Check sheet for the drawn part. Datum: minimum x, y, z corner. Units: mm. A direction names the side the tool comes from. Coordinates: 2 decimals unless noted, no trailing zeros. Order: outer loops, then holes, each group sorted by start corner. A loop starts at its lowest first (then second) coordinate and runs counter-clockwise, first axis right, second up. Notation, with made-up numbers: M 51,58.5 L 75,58.5 A30 cw 75,85.5 Z; hole C 24.25,-29.75 d9. An arc over 180 degrees is marked long. Return JSON: item names as keys, results as strings. Group by question number.
Q1. Go/stop test with flat-tipped pins: pin 1 Ø4 at (y, z) = (32.5, 13) entering from -X; pin 2 Ø0.8 at (x, y) = (30.5, 20.5) entering from -Z; pin 3 Ø8 at (x, y) = (33.5, 28.5) entering from +Z; pin 4 Ø3 at (y, z) = (23, 14) entering from +X. Record where each tip stops, or that it passes through.
Q2. Section check B-B, the plane x = 21. Enter the section's corners in (y, z).
Q3. Thickness scan on probe 1 along Y at (x, z) = (21, 20.4); probe 2 along Z at (x, y) = (12, 25); probe 3 along Y at (x, z) = (25.5, 4). Record the ranges inside material, lowest first.
Q4. Access from +Z, -Z, +X, -X, +Y, -Y to the whole of each face (thin tool, end or side, straight path). Record for the marked faces 1 and 2.
Q5. Section check D-D, the plane z = 9.5. Enter the section's corners in (x, y), then the cut area to 3 significant figures.
Q6. Mould release check, pull along X, two halves, no side actions. Record for the marked faces 3, 4 and 5: pulls with the +X half, pulls with the -X half, needs draft (parallel to the pull), parting line crosses it, or undercut.
Q7. Section check C-C, the plane y = 21. Enter the section's corners in (x, z).
Q8. Section check A-A, the plane z = 1.75. Enter the section's corners in (x, y), then the cut area to 3 significant figures.
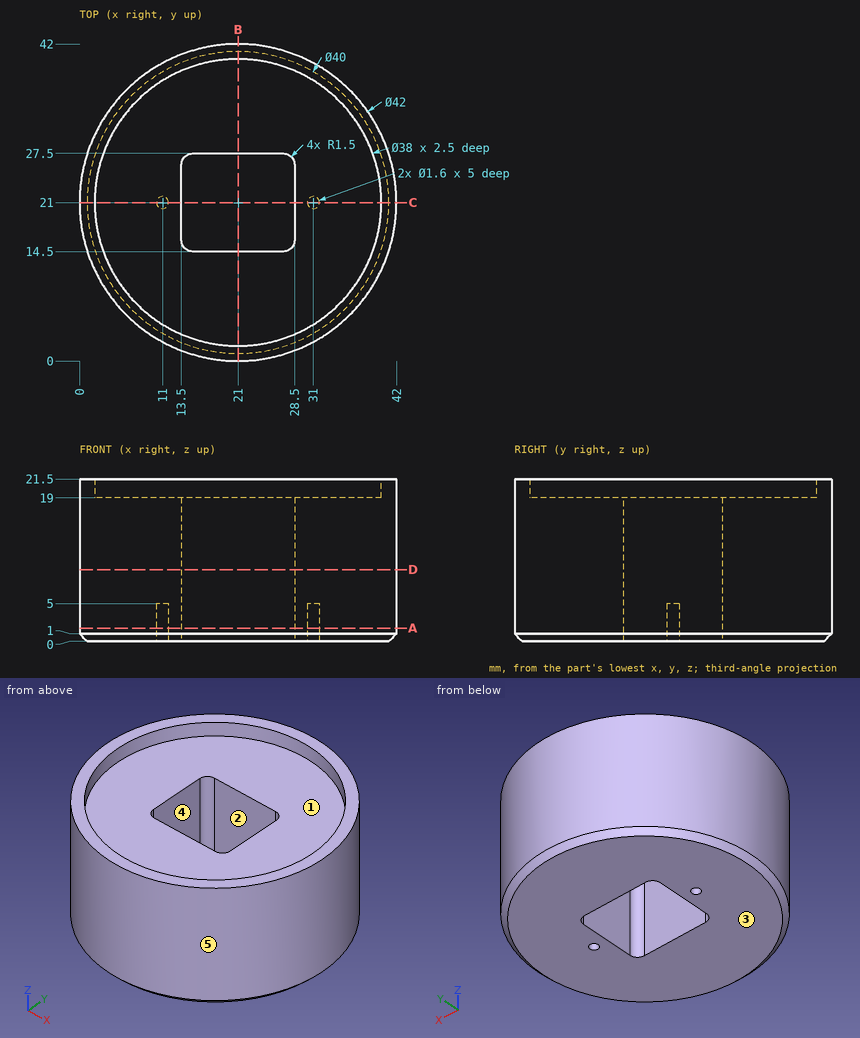
Numbers:
{
 "1": {"pin 1": "stops at x = 2.27", "pin 2": "stops at z = 0", "pin 3": "stops at z = 19", "pin 4": "stops at x = 41.99"},
 "2": {"outline": "M 0,1 L 1,0 L 14.5,0 L 14.5,19 L 2,19 L 2,21.5 L 0,21.5 Z; M 27.5,0 L 41,0 L 42,1 L 42,21.5 L 40,21.5 L 40,19 L 27.5,19 Z"},
 "3": {"probe 1": "y = 0 to 2, 40 to 42", "probe 2": "z = 0 to 19", "probe 3": "y = 0.49 to 14.5, 27.5 to 41.51"},
 "4": {"face 1": "+Z", "face 2": "+Z, -Z"},
 "5": {"outline": "C 21,21 d42; hole M 13.5,16 A1.5 ccw 15,14.5 L 27,14.5 A1.5 ccw 28.5,16 L 28.5,26 A1.5 ccw 27,27.5 L 15,27.5 A1.5 ccw 13.5,26 Z", "area": "1,190 mm2"},
 "6": {"face 3": "needs draft", "face 4": "undercut", "face 5": "parting line crosses it"},
 "7": {"outline": "M 0,1 L 1,0 L 10.2,0 L 10.2,5 L 11.8,5 L 11.8,0 L 13.5,0 L 13.5,19 L 2,19 L 2,21.5 L 0,21.5 Z; M 28.5,0 L 30.2,0 L 30.2,5 L 31.8,5 L 31.8,0 L 41,0 L 42,1 L 42,21.5 L 40,21.5 L 40,19 L 28.5,19 Z"},
 "8": {"outline": "C 21,21 d42; hole C 11,21 d1.6; hole M 13.5,16 A1.5 ccw 15,14.5 L 27,14.5 A1.5 ccw 28.5,16 L 28.5,26 A1.5 ccw 27,27.5 L 15,27.5 A1.5 ccw 13.5,26 Z; hole C 31,21 d1.6", "area": "1,190 mm2"}
}
